from build123d import *

# Parameters (mm, degrees)
F0_R     = 2.5
F1_DEPTH = 3
F2_R     = 1.5
F4_DEPTH = 1.5


with BuildPart() as f1:
    # F0 (on Front) → F1 (new body)
    with BuildSketch(Plane.XZ):
        Circle(F0_R)
    extrude(amount=F1_DEPTH)

    # F2
    f2_edges = [f1.edges().sort_by_distance(p)[0] for p in [
        (-2.5, -3, 0),
    ]]
    fillet(f2_edges, radius=F2_R)

    # F3 (on Front) → F4 (join)
    with BuildSketch(Plane.XZ):
        with BuildLine():
            Line((-10.973479, 10.002215), (-2.837275, 0.974612))
            ThreePointArc((-2.837275, 0.974612), (0.20759, -2.992809), (2.675548, 1.356998))
            Line((2.675548, 1.356998), (16.424086, 15.161496))
            Line((16.424086, 15.161496), (1.566229, 2.558696))
            ThreePointArc((1.566229, 2.558696), (0.188675, 2.994061), (-1.232635, 2.73507))
            Line((-1.232635, 2.73507), (-10.973479, 10.002215))
        make_face()
    extrude(amount=F4_DEPTH)


solid = f1.part
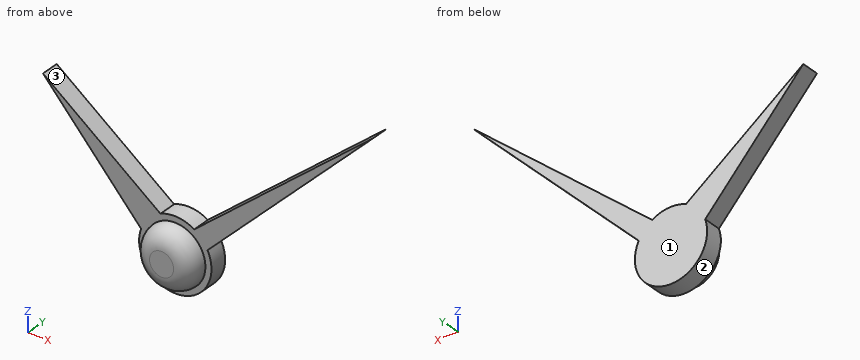
For this review, take the finished solid that the model builds, in its own axes (mm). Face numbers are marked on the shaded views. Give positions to 0.01 mm unless a question says otherwise; leave off trailing zeros. Loops run counter-clockwise (first coordinate to the right, second up) from the corner with the lowest first, then second, coordinate; pieces in that order, holes last. Notation, with made-up numbers: M 14.5,65.25 L 58.5,65.25 A27 ccw 58.5,83.25 Z; hole C 19.5,72 d5. An arc over 180 degrees is marked long. Answer as a JSON object with one key per item and string values. Group by question number.
Q1. Add section A-A on z = 8.25. Give the boundary of the cut face in (x, y).
Q2. Add section D-D on z = 11. Give the boundary of the cut face in (x, y), and give its area (3 significant figures).
Q3. Add section B-B on z = 6. Give the boundary of the cut face in (x, y).
Q4. For probe 1 along Y at (x, z) = (9, 8.75); probe 2 along X at (y, z) = (-0.2, 8); probe 3 along X at (y, z) = (-1.2, 6.75), list the stretches that pass through material, from the lowest coordinate up. Write a range as [from, to].
Q5. Add section C-C on x = -6. Give the boundary of the cut face in (y, z).
Q6. Mouldability with a two-part tool opening along Z and no side actions: class the marked faces 1, 2 and 3 as +Z half, -Z half, draft (parallel to the pull), parting line (faces both ways), or undercut.
Checked values:
{
 "1": {"outline": "M -9.39,-1.5 L -8.62,-1.5 L -8.62,0 L -9.39,0 Z; M 8.28,-1.5 L 9.54,-1.5 L 9.54,0 L 8.28,0 Z"},
 "2": {"outline": "M 11.52,-1.5 L 12.28,-1.5 L 12.28,0 L 11.52,0 Z", "area": "1.14 mm²"},
 "3": {"outline": "M -7.37,-1.5 L -5.61,-1.5 L -5.61,0 L -7.37,0 Z; M 5.62,-1.5 L 7.3,-1.5 L 7.3,0 L 5.62,0 Z"},
 "4": {"probe 1": "[-1.5, 0]", "probe 2": "[-9.17, -8.29], [7.98, 9.29]", "probe 3": "[-8.04, -6.61], [6.51, 8.05]"},
 "5": {"outline": "M -1.5,4.48 L 0,4.48 L 0,6.29 L -1.5,6.29 Z"},
 "6": {"face 1": "draft", "face 2": "undercut", "face 3": "+Z half"}
}
